The listing builds one solid part. Answer for the finished solid, in the listing's coordinates (mm). A direction names the side the tool comes from. Round coordinates to 2 decimals unless told otherwise and drop trailing zeros. Write each loop counter-clockwise with the first axis right and the second up, starting at its lowest first coordinate (ties: lowest second). Pieces come first, ordered by that corner, then holes.
Autodesk Inventor part; units mm, degrees
ref_plane "YZ Plane" through (0, 0, 0) normal (1, 0, 0) x (0, 1, 0)
ref_plane "XZ Plane" through (0, 0, 0) normal (0, 1, 0) x (-1, 0, 0)
sketch "Sketch1" plane through (0, 0, 0) normal (0, 1, 0) x (-1, 0, 0)
  line L0 (0, 0) -> (-28, 0)
  line L1 (-28, 0) -> (-28, 16)
  line L2 (-28, 16) -> (0, 16)
  line L3 (0, 16) -> (0, 0)
  circle A0 centre (-25.1, 13.15) radius 1.5
  circle A1 centre (-2.9, 2.85) radius 1.5
  line L4 (-28, 8) -> (0, 8) construction
  line L5 (-14, 0) -> (-14, 16) construction
  line L6 (-25.1, 13.15) -> (-28, 13.15) construction
  line L7 (-25.1, 13.15) -> (-25.1, 16) construction
  line L8 (-2.9, 2.85) -> (-2.9, 0) construction
  line L9 (-2.9, 2.85) -> (0, 2.85) construction
  dimension "d0" = 28
  dimension "d1" = 16
  dimension "d2" = 3
  dimension "d3" = 3
  dimension "d4" = 22.2
  dimension "d5" = 10.3
extrude "Extrusion1" add sketch "Sketch1" along normal blind 10.2
ref_plane "Work Plane1" through (0, 0, 4.5) normal (0, 0, 1) x (1, 0, 0)
sketch "Sketch2" plane through (0, 0, 4.5) normal (0, 0, 1) x (1, 0, 0)
  line L0 (28, 1.925) -> (33.5, 1.925)
  line L1 (33.5, 1.925) -> (33.5, 2.8)
  line L2 (33.5, 8.275) -> (28, 8.275)
  line L3 (28, 8.275) -> (28, 1.925)
  line L4 (33.5, 7.4) -> (40, 7.4)
  line L5 (40, 7.4) -> (40, 2.8)
  line L6 (40, 2.8) -> (33.5, 2.8)
  line L7 (33.5, 7.4) -> (33.5, 8.275)
  line L8 (33.5, 2.8) -> (33.5, 7.4) construction
  line L9 (28, 1.925) -> (28, 0) construction
  line L10 (28, 8.275) -> (28, 10.2) construction
  circle A0 centre (38, 5.1) radius 0.85
  line L11 (38, 5.1) -> (38, 2.8) construction
  line L12 (38, 7.4) -> (38, 5.1) construction
  point P0 (0, 0)
  dimension "d12" = 6.5
  dimension "d13" = 1.7
  dimension "d14" = 2
  dimension "d15" = 12
  dimension "d16" = 4.6
  dimension "d17" = 6.35
extrude "Extrusion2" add sketch "Sketch2" along normal blind 0.8
ref_plane "Work Plane2" through (0, 1, 0) normal (0, -1, 0) x (1, 0, 0)
sketch "Sketch4" plane through (0, 1, 0) normal (0, -1, 0) x (1, 0, 0)
  line L0 (16.8061, 0) -> (16, 0)
  line L1 (16, 0) -> (16, -2.2)
  line L2 (16.8, -3) -> (16.8, -3)
  line L3 (16.8, -3) -> (26.1061, -3)
  line L4 (26.1061, -3) -> (26.1061, -2.2)
  line L5 (26.1061, -2.2) -> (17.6061, -2.2)
  line L6 (16.8061, -1.4) -> (16.8061, 0)
  arc A0 (16, -2.2) -> (16.8, -3) centre (16.8, -2.2) ccw
  arc A1 (16.8061, -1.4) -> (17.6061, -2.2) centre (17.6061, -1.4) ccw
  line L7 (0, 0) -> (0, 16)
  point P0 (16, -3)
  point P1 (16.8061, -2.2)
  dimension "d32" = 0.8
  dimension "d33" = 3
  dimension "d34" = 9.3
  dimension "d35" = 0.8
  dimension "d36" = 0.8
  dimension "d41" = 16
extrude "Extrusion3" add sketch "Sketch4" against normal blind 8.5
sketch "Sketch5" plane through (0, 1, 0) normal (0, -1, 0) x (1, 0, 0)
  line L0 (28, 16) -> (0, 16)
  line L1 (17.8, 16) -> (17, 16)
  line L2 (17, 16) -> (17, 17.5509)
  line L3 (17, 19) -> (17.8, 19) construction
  line L4 (17.8, 18.2775) -> (17.8, 16)
  line L5 (0, 0) -> (0, 16)
  line L6 (17.0813, 19.0734) -> (-10.6, 21.9)
  line L7 (-10.6817, 21.1) -> (-10.6, 21.9)
  line L8 (-10.6817, 21.1) -> (16.2813, 18.3467)
  line L9 (26.1061, -3) -> (16.8, -3)
  line L10 (40, 4.5) -> (40, 5.3)
  line L11 (17, 18.2733) -> (17, 19) construction
  arc A0 (17, 17.5509) -> (16.2813, 18.3467) centre (16.2, 17.5509) ccw
  arc A1 (17.8, 18.2775) -> (17.0813, 19.0734) centre (17, 18.2775) ccw
  dimension "d44" = 0.8
  dimension "d45" = 3
  dimension "d46" = 17
  dimension "d48" = 0.8
  dimension "d49" = 24.9
  dimension "d50" = 50.6
  dimension "d51" = 0.8
ref_plane "Work Plane4" through (0, 5.6, 0) normal (0, -1, 0) x (1, 0, 0)
sketch "Sketch6" plane through (0, 5.6, 0) normal (0, -1, 0) x (1, 0, 0)
  line L0 (17.8, 16) -> (17, 16)
  line L1 (17, 16) -> (17, 17.5509)
  line L2 (17, 19) -> (17.8, 19) construction
  line L3 (17.8, 18.2775) -> (17.8, 16)
  line L4 (17.0813, 19.0734) -> (-10.6, 21.9)
  line L5 (-10.6817, 21.1) -> (-10.6, 21.9)
  line L6 (-10.6817, 21.1) -> (16.2813, 18.3467)
  line L7 (17, 18.2733) -> (17, 19) construction
  arc A0 (17, 17.5509) -> (16.2813, 18.3467) centre (16.2, 17.5509) ccw
  arc A1 (17.8, 18.2775) -> (17.0813, 19.0734) centre (17, 18.2775) ccw
  line L8 (40, 4.5) -> (40, 5.3)
  line L9 (16.8, -3) -> (26.1061, -3)
  line L10 (0, 16) -> (0, 0)
  dimension "d54" = 0.8
  dimension "d55" = 3
  dimension "d57" = 0.8
  dimension "d60" = 0.8
  dimension "d61" = 50.6
  dimension "d62" = 24.9
  dimension "d63" = 17
extrude "Extrusion5" add sketch "Sketch6" along normal mid plane 4.35
properties part number "game-switch"
1. Given pin 1 (12 mm diameter, centred on x = 26, z = 10, fed in from -Y); pin 2 (1.2 mm diameter, centred on y = 4.5, z = 16.5, fed in from -X); pin 3 (2.5 mm diameter, centred on y = 5, z = -1.5, fed in from -X); pin 4 (6 mm diameter, centred on x = -3.5, y = 1.5, fed in from +Z), each flat-ended and moving along its own axis, determine where each tip first touches the part or whether it passes through.
Geometry says:
pin 1: stops at y = 0
pin 2: stops at x = 0
pin 3: stops at x = 16
pin 4: stops at z = 21.41
2. Section D-D on z = 13.15 is taken. Determine the outline of the cut face in (x, y), plus the area to 3 significant figures.
Geometry says:
outline: (0, 0) - (23.6, 0) - (23.6, 10.2) - (0, 10.2) - close; (26.6, 0) - (28, 0) - (28, 10.2) - (26.6, 10.2) - close
area: 255 mm2
3. A tool of negligible diameter and unlimited length cuts with its end or side. For faces 4 (the face through (20.3, 9.5, -2.4)), 5 (the face through (0, 5, 8)), 6 (the face through (5, 7.775, 20)), from which of +Z, -Z, +X, -X, +Y, -Y can it reach the whole face along a straight path? Write none if from no direction.
Geometry says:
face 4: -Z, +X, -X, +Y
face 5: -Z, -X, +Y, -Y
face 6: +Z, +X, -X, +Y
4. Section A-A on x = 38 is taken. Determine the outline of the cut face in (y, z).
Geometry says:
outline: (2.8, 4.5) - (4.25, 4.5) - (4.25, 5.3) - (2.8, 5.3) - close; (5.95, 4.5) - (7.4, 4.5) - (7.4, 5.3) - (5.95, 5.3) - close
5. Section B-B on y = 5.1 is taken. Give the number of separate pieces and of enclosed holes in the cut face, plus the area to 3 significant figures.
Geometry says:
separate pieces: 2
enclosed holes: 2
area: 477 mm2
6. Section C-C on x = 25.1 is taken. Determine the outline of the cut face in (y, z), plus the area to 3 significant figures.
Geometry says:
outline: (0, 0) - (10.2, 0) - (10.2, 11.65) - (0, 11.65) - close; (0, 14.65) - (10.2, 14.65) - (10.2, 16) - (0, 16) - close; (1, -3) - (9.5, -3) - (9.5, -2.2) - (1, -2.2) - close
area: 139 mm2
7. Straight lines are drawn through the part: line 1 along Z through (x, y) = (25.1, 4.5); line 2 along Y through (x, z) = (38, 5.05); line 3 along Z through (x, y) = (3, 1). For each, find the intervals that lie inside material, in ascending order.
Geometry says:
line 1: z = -3 to -2.2, 0 to 11.65, 14.65 to 16
line 2: y = 2.8 to 4.25, 5.95 to 7.4
line 3: z = 0 to 1.35, 4.35 to 16
8. For a pull along Z with two mould halves and no side action, classify faces 1 (the face through (28, 5, 8)), 2 (the face through (3.434, 5.63, 20.467)), 3 (the face through (1.514, 5.029, 3.425)) as released by +Z, released by -Z, zero draft, split by the parting line, or undercut.
Geometry says:
face 1: zero draft
face 2: released by +Z
face 3: undercut
